Can you work these out from the model? Positions are in its coordinate system, mm. A direction names the side the tool comes from. Give positions to 0.01 mm unless a question says otherwise; leave off trailing zeros. Write each loop counter-clockwise with the first axis right and the second up, starting at its lowest first coordinate (ties: lowest second). Pieces come first, ordered by that corner, then holes. Notation, with made-up numbers: M 48.5,69 L 104.5,69 A25 cw 104.5,107 Z; hole C 55,7 d1. An arc over 180 degrees is marked long. Write each question's results on one line, items separated by ' | '.
from build123d import *

# Parameters (mm, degrees)
ESQUISSE1_W        = 105
ESQUISSE1_H        = 105
ESQUISSE1_R        = 4.25
ESQUISSE1_R_2      = 3.25
ESQUISSE1_R_3      = 2
BOSS_EXTRU_1_DEPTH = 1
ESQUISSE1_4_R      = 4.25
ESQUISSE1_4_R_2    = 3.25
BOSS_EXTRU_3_DEPTH = 2
CONG_1_R           = 5


with BuildPart() as part:
    # Esquisse1 → Boss.-Extru.1 (new body)
    # profile 1 of 5: a face of its own
    with BuildSketch(Plane.XY):
        Rectangle(ESQUISSE1_W, ESQUISSE1_H)
        with Locations((-43.75, 46)):
            Circle(ESQUISSE1_R, mode=Mode.SUBTRACT)
        with Locations((46, -43.75)):
            Circle(ESQUISSE1_R, mode=Mode.SUBTRACT)
    # profile 2 of 5: a face of its own
    with BuildSketch(Plane.XY):
        with Locations((-43.75, 46)):
            Circle(ESQUISSE1_R)
        with Locations((-43.75, 46)):
            Circle(ESQUISSE1_R_2, mode=Mode.SUBTRACT)
    # profile 3 of 5: a face of its own
    with BuildSketch(Plane.XY):
        with Locations((-43.75, 46)):
            Circle(ESQUISSE1_R_2)
        with Locations((-43.75, 46)):
            Circle(ESQUISSE1_R_3, mode=Mode.SUBTRACT)
    # profile 4 of 5: a face of its own
    with BuildSketch(Plane.XY):
        with Locations((46, -43.75)):
            Circle(ESQUISSE1_R)
        with Locations((46, -43.75)):
            Circle(ESQUISSE1_R_2, mode=Mode.SUBTRACT)
    # profile 5 of 5: a face of its own
    with BuildSketch(Plane.XY):
        with Locations((46, -43.75)):
            Circle(ESQUISSE1_R_2)
        with Locations((46, -43.75)):
            Circle(ESQUISSE1_R_3, mode=Mode.SUBTRACT)
    extrude(amount=BOSS_EXTRU_1_DEPTH)

    # Esquisse1_4 → Boss.-Extru.3 (add)
    # profile 1 of 2: a face of its own
    with BuildSketch(Plane.XY):
        with Locations((-43.75, 46)):
            Circle(ESQUISSE1_4_R)
        with Locations((-43.75, 46)):
            Circle(ESQUISSE1_4_R_2, mode=Mode.SUBTRACT)
    # profile 2 of 2: a face of its own
    with BuildSketch(Plane.XY):
        with Locations((46, -43.75)):
            Circle(ESQUISSE1_4_R)
        with Locations((46, -43.75)):
            Circle(ESQUISSE1_4_R_2, mode=Mode.SUBTRACT)
    extrude(amount=BOSS_EXTRU_3_DEPTH)

    # Cong_1
    cong_1_edges = [part.edges().sort_by_distance(p)[0] for p in [
        (52.5, -52.5, 0.5),
        (-52.5, -52.5, 0.5),
        (-52.5, 52.5, 0.5),
        (52.5, 52.5, 0.5),
    ]]
    fillet(cong_1_edges, radius=CONG_1_R)


solid = part.part
Item 1: I want a section at B-B, the plane x = 46. Please give me the cut outline in (y, z).
Geometry says:
outline: M -52.5,0 L -45.75,0 L -45.75,1 L -47,1 L -47,2 L -48,2 L -48,1 L -52.5,1 Z; M -41.75,0 L 52.5,0 L 52.5,1 L -39.5,1 L -39.5,2 L -40.5,2 L -40.5,1 L -41.75,1 Z
Item 2: If I drill on line 1 (Y direction, x = -43.75, z = 0.4); line 2 (X direction, y = 46, z = 1.55); line 3 (Y direction, x = -43.75, z = 1.5), over which ranges is the centre line in solid material (lowest first)? Write a range as from..to.
Geometry says:
line 1: y = -52.5..44, 48..52.5 | line 2: x = -48..-47, -40.5..-39.5 | line 3: y = 41.75..42.75, 49.25..50.25
Item 3: I'm going to push a flat-ended pin straight in: pin 1 (3 mm diameter, centred on x = -44.5, y = 46.5, fed in from +Z). Where does the tip first touch, or does it pass through?
Geometry says:
pin 1: stops at z = 1
Item 4: I want a section at C-C, the plane z = 1.5. Please give me the cut outline in (x, y), and give its area (3 significant figures).
Geometry says:
outline: C -43.75,46 d8.5; C 46,-43.75 d8.5; hole C -43.75,46 d6.5; hole C 46,-43.75 d6.5 | area: 47.1 mm2
Item 5: Thinking about a two-plate mould opening in Y: for faces 3 (the face through (45, -47, 2)), 4 (the face through (-41.6, 45.3, 1)), 5 (the face through (-51.07, 51, 0.51)), which applies, +Y half, -Y half, draft (parallel to the pull), parting line (faces both ways), or undercut?
Geometry says:
face 3: draft | face 4: undercut | face 5: +Y half
Item 6: I want a section at A-A, the plane y = -43.75. Please give me the cut outline in (x, z), and give its area (3 significant figures).
Geometry says:
outline: M -52.5,0 L 44,0 L 44,1 L 42.75,1 L 42.75,2 L 41.75,2 L 41.75,1 L -52.5,1 Z; M 48,0 L 52.5,0 L 52.5,1 L 50.25,1 L 50.25,2 L 49.25,2 L 49.25,1 L 48,1 Z | area: 103 mm2
Item 7: For faces 1 (the face through (46, -46, 1)), 2 (the face through (51, 51.07, 0.51)), which set-ups out of +Z, -Z, +X, -X, +Y, -Y let a thin tool reach every point of the face, with its end or its side?
Geometry says:
face 1: +Z | face 2: +Z, -Z, +X, +Y
Item 8: I want a section at D-D, the plane y = -5. Please give me the cut outline in (x, z).
Geometry says:
outline: M -52.5,0 L 52.5,0 L 52.5,1 L -52.5,1 Z
